Answer from the drawing. Dimensions are ordinates in mm from the lowest x, y and z of the part. Coordinates: 2 decimals unless noted, no trailing zeros. Write each loop counter-clockwise with the first axis right and the second up, starting at its lowest first coordinate (ties: lowest second). Pieces come first, ordered by that corner, then holes.
(1) Section C-C on z = 118.5 is taken. Write down the section's boundary in (x, y).
(2) Section B-B on x = 90.5 is taken. Write down the section's boundary in (y, z).
(3) Section A-A on y = 8 is taken. Write down the section's boundary in (x, z) (1 decimal).
(4) Given pin 1 (3 mm diameter, centred on y = 6.5, z = 121.5, fed in from +X) (1 decimal), flat-ended and moving along its own axis, determine where the tip first touches the part or whether it passes through.
(5) Find the intervals of material crossed by probe 1 along Z at (x, y) = (71.5, 3.5) (1 decimal); probe 2 along Z at (x, y) = (124.5, 1.5) (1 decimal); probe 3 along X at (y, z) = (11, 98.5), in increasing order.
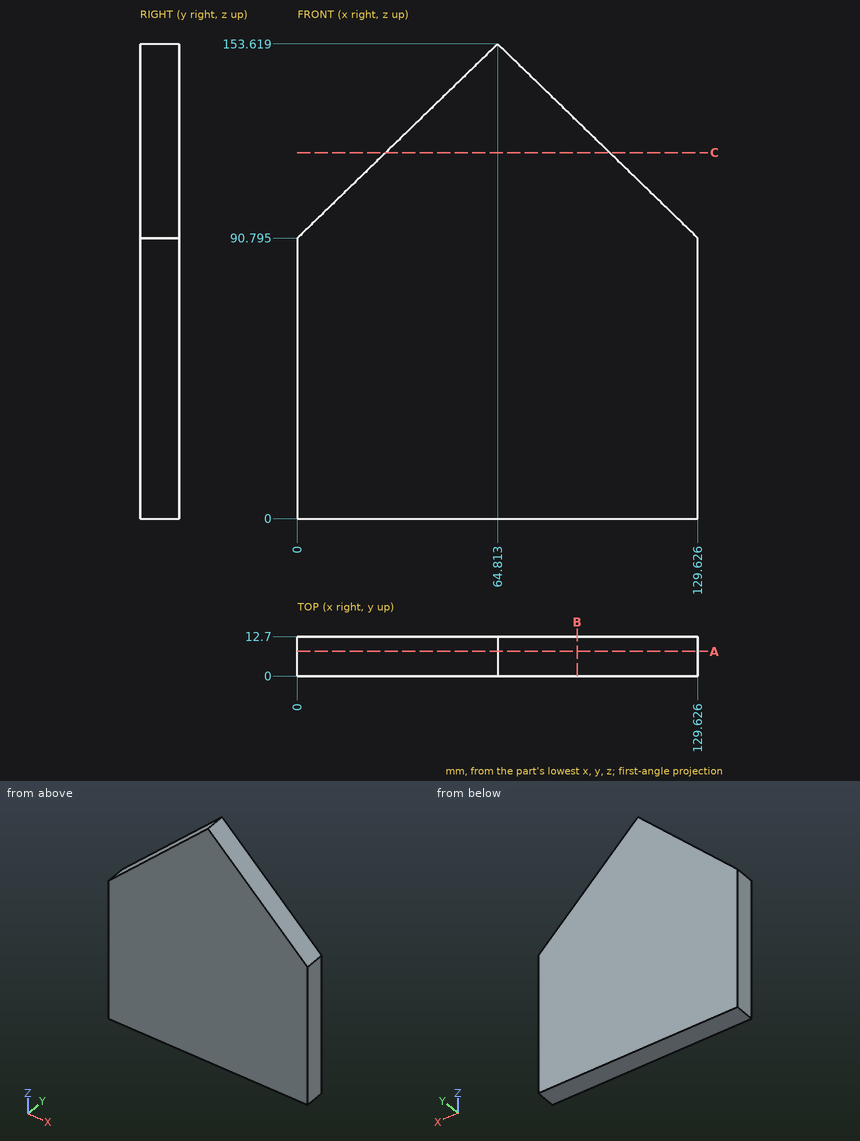
Response:
1. outline: (28.58, 0) - (101.04, 0) - (101.04, 12.7) - (28.58, 12.7) - close
2. outline: (0, 0) - (12.7, 0) - (12.7, 128.72) - (0, 128.72) - close
3. outline: (0, 0) - (129.6, 0) - (129.6, 90.8) - (64.8, 153.6) - (0, 90.8) - close
4. pin 1: stops at x = 99.5
5. probe 1: z = 0 to 147.1
5. probe 2: z = 0 to 95.8
5. probe 3: x = 7.95 to 121.68
